Read the model definition and answer for the solid it produces. Units are mm, in the model's axes. Face numbers are marked on the shaded views. A direction names the side the tool comes from. Coordinates: 2 decimals unless noted, no trailing zeros. Order: outer loops, then holes, each group sorted by start corner. A loop starts at its lowest first (then second) coordinate and runs counter-clockwise, first axis right, second up. Notation, with made-up numbers: M -27.75,-36.75 L 24.25,-36.75 A9 ccw 24.25,-25.75 Z; hole C -9,-32 d7. An arc over 180 degrees is marked long. Write each question's results on one line, items separated by ' | '.
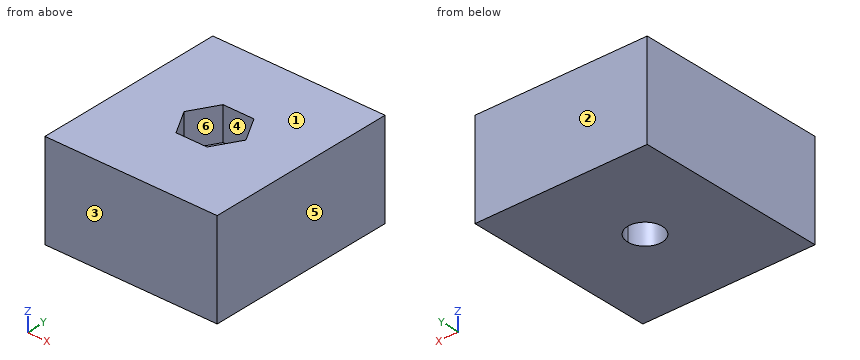
```python
from build123d import *

# Parameters (mm, degrees)
SKETCH1_W           = 18
SKETCH1_H           = 20
BOSS_EXTRUDE1_DEPTH = 10
CUT_EXTRUDE1_DEPTH  = 17.763054614
CUT_EXTRUDE2_DEPTH  = 3.5


with BuildPart() as part:
    # Sketch1 → Boss-Extrude1 (new body)
    with BuildSketch(Plane.XY):
        Rectangle(SKETCH1_W, SKETCH1_H)
    extrude(amount=BOSS_EXTRUDE1_DEPTH)

    # Sketch2 → Cut-Extrude1 (cut, through all)
    with BuildSketch(Plane.XY.offset(10)):
        with BuildLine():
            ThreePointArc((1.8, 0), (1.644300114, 0.732309453), (1.204136517, 1.337929463))
            Line((1.204136517, 1.337929463), (-1.204136517, -1.337929463))
            ThreePointArc((-1.204136517, -1.337929463), (0.732309453, -1.644300114), (1.8, 0))
        make_face()
        with BuildLine():
            Line((-1.204136517, -1.337929463), (1.204136517, 1.337929463))
            ThreePointArc((1.204136517, 1.337929463), (-1.337929463, 1.204136517), (-1.204136517, -1.337929463))
        make_face()
    extrude(amount=-CUT_EXTRUDE1_DEPTH, mode=Mode.SUBTRACT)

    # Sketch3 → Cut-Extrude2 (cut)
    with BuildSketch(Plane.XY.offset(10)):
        Polygon((1.616580754, 2.8), (-1.616580754, 2.8), (-3.233161507, 0), (-1.616580754, -2.8), (1.616580754, -2.8), (3.233161507, 0), align=None)
    extrude(amount=-CUT_EXTRUDE2_DEPTH, mode=Mode.SUBTRACT)


solid = part.part
```
(1) The part is cut by section A-A, the plane z = 1.75. Write down the section's boundary in (x, y).
Conclusion:
outline: M -9,-10 L 9,-10 L 9,10 L -9,10 Z; hole C 0,0 d3.6
(2) The mould has two halves that part along Y. Classify the marked faces 1, 2, 3 and 4: pulls with the +Y half, pulls with the -Y half, needs draft (parallel to the pull), parting line crosses it, or undercut.
Conclusion:
face 1: needs draft | face 2: pulls with the +Y half | face 3: pulls with the -Y half | face 4: undercut
(3) The part is cut by section B-B, the plane x = 0. Write down the section's boundary in (y, z), then the cut area to 3 significant figures.
Conclusion:
outline: M -10,0 L -1.8,0 L -1.8,6.5 L -2.8,6.5 L -2.8,10 L -10,10 Z; M 1.8,0 L 10,0 L 10,10 L 2.8,10 L 2.8,6.5 L 1.8,6.5 Z | area: 157 mm²
(4) Straight lines are drawn through the part: line 1 (Y direction, x = 1, z = 8.5); line 2 (Y direction, x = -0.25, z = 4.5); line 3 (X direction, y = -1, z = 2.75). For each, find the intervals that lie inside material, in ascending order.
Conclusion:
line 1: -10 to -2.8, 2.8 to 10 | line 2: -10 to -1.78, 1.78 to 10 | line 3: -9 to -1.5, 1.5 to 9
(5) For the marked faces 5 and 6, determine the directions among +Z, -Z, +X, -X, +Y, -Y from which every point of the face is accessible in a straight line to the end or side of a thin tool.
Conclusion:
face 5: +Z, -Z, +X, +Y, -Y | face 6: +Z
